```python
from build123d import *

# Parameters (mm, degrees)
MAIN_WEB_PROFILE_W                      = 60
MAIN_WEB_PROFILE_H                      = 14
MAIN_WEB_DEPTH                          = 4
SHOULDER_HORN_FLANGE_PROFILE_R          = 16
SHOULDER_HORN_FLANGE_DEPTH              = 4
ELBOW_SERVO_MOUNT_PROFILE_W             = 48
ELBOW_SERVO_MOUNT_PROFILE_H             = 28
ELBOW_SERVO_MOUNT_DEPTH                 = 4
SG90_BODY_CLEARANCE_START               = -5
SG90_BODY_CLEARANCE_PROFILE_W           = 23.8
SG90_BODY_CLEARANCE_PROFILE_H           = 13
SG90_BODY_CLEARANCE_DEPTH               = 97.49863387
ELBOW_TAB_FASTENERS_START               = -50
ELBOW_TAB_FASTENERS_PROFILE_R           = 1.3
ELBOW_TAB_FASTENERS_DEPTH               = 142.49863387
SHOULDER_CENTER_SCREW_ACCESS_START      = -50
SHOULDER_CENTER_SCREW_ACCESS_PROFILE_R  = 4
SHOULDER_CENTER_SCREW_ACCESS_DEPTH      = 142.49863387
CABLE_TIE_HOLES_START                   = -50
CABLE_TIE_HOLES_PROFILE_R               = 1.6
CABLE_TIE_HOLES_DEPTH                   = 142.49863387
PASSIVE_LOWER_MOUNT_BOSS_PROFILE_R      = 5
PASSIVE_LOWER_MOUNT_BOSS_DEPTH          = 4
PASSIVE_UPPER_MOUNT_BOSS_PROFILE_R      = 5
PASSIVE_UPPER_MOUNT_BOSS_DEPTH          = 4
PASSIVE_CHEEK_STANDOFFS_START           = -50
PASSIVE_CHEEK_STANDOFFS_PROFILE_R       = 1.6
PASSIVE_CHEEK_STANDOFFS_DEPTH           = 142.49863387
SHOULDER_DOWEL_SUPPORT_HUB_START        = 4
SHOULDER_DOWEL_SUPPORT_HUB_PROFILE_R    = 7
SHOULDER_DOWEL_SUPPORT_HUB_PROFILE_R_2  = 4
SHOULDER_DOWEL_SUPPORT_HUB_DEPTH        = 4
RAISED_M3_WASHER_SEATS_HEIGHT8_START    = 4
RAISED_M3_WASHER_SEATS_PCD14_PROFILE_R  = 3.5
RAISED_M3_WASHER_SEATS_HEIGHT8_DEPTH    = 4
METAL_HORN_M3_CLEARANCE_PCD14_START     = -50
METAL_HORN_M3_CLEARANCE_PCD14_PROFILE_R = 1.6
METAL_HORN_M3_CLEARANCE_PCD14_DEPTH     = 142.760557976
RESTORE_SHOULDER_SLEEVE_BORE_START      = -50
RESTORE_SHOULDER_SLEEVE_BORE_PROFILE_R  = 4
RESTORE_SHOULDER_SLEEVE_BORE_DEPTH      = 142.760557976
FILLET1_R                               = 7.5


with BuildPart() as part:
    # Main_web_profile → Main_web (new body)
    with BuildSketch(Plane.XY):
        with Locations((30, 0)):
            Rectangle(MAIN_WEB_PROFILE_W, MAIN_WEB_PROFILE_H)
    extrude(amount=MAIN_WEB_DEPTH)

    # Shoulder_horn_flange_profile → Shoulder_horn_flange (add)
    with BuildSketch(Plane.XY):
        Circle(SHOULDER_HORN_FLANGE_PROFILE_R)
    extrude(amount=SHOULDER_HORN_FLANGE_DEPTH)

    # Elbow_servo_mount_profile → Elbow_servo_mount (add)
    with BuildSketch(Plane.XY):
        with Locations((66, 0)):
            Rectangle(ELBOW_SERVO_MOUNT_PROFILE_W, ELBOW_SERVO_MOUNT_PROFILE_H)
    extrude(amount=ELBOW_SERVO_MOUNT_DEPTH)

    # SG90_body_clearance_profile → SG90_body_clearance (cut, through all)
    with BuildSketch(Plane.XY.offset(SG90_BODY_CLEARANCE_START)):
        with Locations((65.5, 0)):
            Rectangle(SG90_BODY_CLEARANCE_PROFILE_W, SG90_BODY_CLEARANCE_PROFILE_H)
    extrude(amount=SG90_BODY_CLEARANCE_DEPTH, mode=Mode.SUBTRACT)

    # Elbow_tab_fasteners_profile → Elbow_tab_fasteners (cut, through all)
    with BuildSketch(Plane.XY.offset(ELBOW_TAB_FASTENERS_START)):
        with Locations(Location((51, 0, 0), (0, 0, 180))):
            Circle(ELBOW_TAB_FASTENERS_PROFILE_R)
        with Locations(Location((80, 0, 0), (0, 0, 180))):
            Circle(ELBOW_TAB_FASTENERS_PROFILE_R)
    extrude(amount=ELBOW_TAB_FASTENERS_DEPTH, mode=Mode.SUBTRACT)

    # Shoulder_center_screw_access_profile → Shoulder_center_screw_access (cut, through all)
    with BuildSketch(Plane.XY.offset(SHOULDER_CENTER_SCREW_ACCESS_START)):
        with Locations(Location((0, 0, 0), (0, 0, 180))):
            Circle(SHOULDER_CENTER_SCREW_ACCESS_PROFILE_R)
    extrude(amount=SHOULDER_CENTER_SCREW_ACCESS_DEPTH, mode=Mode.SUBTRACT)

    # Cable_tie_holes_profile → Cable_tie_holes (cut, through all)
    with BuildSketch(Plane.XY.offset(CABLE_TIE_HOLES_START)):
        with Locations(Location((27, -3, 0), (0, 0, 180))):
            Circle(CABLE_TIE_HOLES_PROFILE_R)
        with Locations(Location((27, 3, 0), (0, 0, 180))):
            Circle(CABLE_TIE_HOLES_PROFILE_R)
    extrude(amount=CABLE_TIE_HOLES_DEPTH, mode=Mode.SUBTRACT)

    # Passive_lower_mount_boss_profile → Passive_lower_mount_boss (add)
    with BuildSketch(Plane.XY):
        with Locations((35, -9)):
            Circle(PASSIVE_LOWER_MOUNT_BOSS_PROFILE_R)
    extrude(amount=PASSIVE_LOWER_MOUNT_BOSS_DEPTH)

    # Passive_upper_mount_boss_profile → Passive_upper_mount_boss (add)
    with BuildSketch(Plane.XY):
        with Locations((35, 9)):
            Circle(PASSIVE_UPPER_MOUNT_BOSS_PROFILE_R)
    extrude(amount=PASSIVE_UPPER_MOUNT_BOSS_DEPTH)

    # Passive_cheek_standoffs_profile → Passive_cheek_standoffs (cut, through all)
    with BuildSketch(Plane.XY.offset(PASSIVE_CHEEK_STANDOFFS_START)):
        with Locations(Location((35, -9, 0), (0, 0, 180))):
            Circle(PASSIVE_CHEEK_STANDOFFS_PROFILE_R)
        with Locations(Location((35, 9, 0), (0, 0, 180))):
            Circle(PASSIVE_CHEEK_STANDOFFS_PROFILE_R)
    extrude(amount=PASSIVE_CHEEK_STANDOFFS_DEPTH, mode=Mode.SUBTRACT)

    # Shoulder_dowel_support_hub_profile → Shoulder_dowel_support_hub (add)
    with BuildSketch(Plane.XY.offset(SHOULDER_DOWEL_SUPPORT_HUB_START)):
        Circle(SHOULDER_DOWEL_SUPPORT_HUB_PROFILE_R)
        with Locations(Location((0, 0, 0), (0, 0, 180))):
            Circle(SHOULDER_DOWEL_SUPPORT_HUB_PROFILE_R_2, mode=Mode.SUBTRACT)
    extrude(amount=SHOULDER_DOWEL_SUPPORT_HUB_DEPTH)

    # Raised_M3_washer_seats_PCD14_profile → Raised_M3_washer_seats_height8 (add)
    with BuildSketch(Plane.XY.offset(RAISED_M3_WASHER_SEATS_HEIGHT8_START)):
        with Locations((7, 0)):
            Circle(RAISED_M3_WASHER_SEATS_PCD14_PROFILE_R)
        with Locations((-7, 0)):
            Circle(RAISED_M3_WASHER_SEATS_PCD14_PROFILE_R)
        with Locations((0, 7)):
            Circle(RAISED_M3_WASHER_SEATS_PCD14_PROFILE_R)
        with Locations((0, -7)):
            Circle(RAISED_M3_WASHER_SEATS_PCD14_PROFILE_R)
    extrude(amount=RAISED_M3_WASHER_SEATS_HEIGHT8_DEPTH)

    # Metal_horn_M3_clearance_PCD14_profile → Metal_horn_M3_clearance_PCD14 (cut, through all)
    with BuildSketch(Plane.XY.offset(METAL_HORN_M3_CLEARANCE_PCD14_START)):
        with Locations(Location((7, 0, 0), (0, 0, 180))):
            Circle(METAL_HORN_M3_CLEARANCE_PCD14_PROFILE_R)
        with Locations(Location((-7, 0, 0), (0, 0, 180))):
            Circle(METAL_HORN_M3_CLEARANCE_PCD14_PROFILE_R)
        with Locations(Location((0, 7, 0), (0, 0, 180))):
            Circle(METAL_HORN_M3_CLEARANCE_PCD14_PROFILE_R)
        with Locations(Location((0, -7, 0), (0, 0, 180))):
            Circle(METAL_HORN_M3_CLEARANCE_PCD14_PROFILE_R)
    extrude(amount=METAL_HORN_M3_CLEARANCE_PCD14_DEPTH, mode=Mode.SUBTRACT)

    # Restore_shoulder_sleeve_bore_profile → Restore_shoulder_sleeve_bore (cut, through all)
    with BuildSketch(Plane.XY.offset(RESTORE_SHOULDER_SLEEVE_BORE_START)):
        with Locations(Location((0, 0, 0), (0, 0, 180))):
            Circle(RESTORE_SHOULDER_SLEEVE_BORE_PROFILE_R)
    extrude(amount=RESTORE_SHOULDER_SLEEVE_BORE_DEPTH, mode=Mode.SUBTRACT)

    # Fillet1
    # the kernel refuses this fillet: 7.5 mm, written as the material it takes off along each edge
    with BuildSketch(Plane(origin=(42, -14, -18.708286934), x_dir=(0, 1, 0), z_dir=(0, 0, 1))) as fillet1_piece_1:
        with BuildLine():
            CenterArc((7.5, -7.483314774), FILLET1_R, 93.822553729, 86.177446271)
            Line((0, -7.483314774), (-0.15, -7.483314774))
            Line((-0.15, -7.483314774), (-0.15, 0))
            Line((-0.15, 0), (0, 0.15))
            ThreePointArc((0, 0.15), (3.5, 0.15), (6.99, 0.149666295))
            Line((6.99, 0.149666295), (7, 0))
        make_face()
    extrude(amount=41.416573868, mode=Mode.SUBTRACT)
    with BuildSketch(Plane(origin=(90, -14, -18.75), x_dir=(-1, 0, 0), z_dir=(0, 0, 1)), Plane(origin=(90, 14, -18.75), x_dir=(0, -1, 0), z_dir=(0, 0, 1))) as fillet1_piece_2:
        with BuildLine():
            CenterArc((FILLET1_R, -FILLET1_R), FILLET1_R, 90, 90)
            Line((0, -FILLET1_R), (-FILLET1_R * 0.02, -FILLET1_R))
            Line((-FILLET1_R * 0.02, -FILLET1_R), (-FILLET1_R * 0.02, FILLET1_R * 0.02))
            Line((-FILLET1_R * 0.02, FILLET1_R * 0.02), (FILLET1_R, FILLET1_R * 0.02))
            Line((FILLET1_R, FILLET1_R * 0.02), (FILLET1_R, 0))
        make_face()
    extrude(amount=41.5, mode=Mode.SUBTRACT)
    with BuildSketch(Plane(origin=(42, 14, -18.708286934), x_dir=(0, -1, 0), z_dir=(0, 0, 1))) as fillet1_piece_3:
        with BuildLine():
            CenterArc((7.5, 7.483314774), FILLET1_R, 180, 86.177446271)
            Line((0, 7.483314774), (-0.15, 7.483314774))
            Line((-0.15, 7.483314774), (-0.15, 0))
            Line((-0.15, 0), (0, -0.15))
            ThreePointArc((0, -0.15), (3.5, -0.15), (6.99, -0.149666295))
            Line((6.99, -0.149666295), (7, 0))
        make_face()
    extrude(amount=41.416573868, mode=Mode.SUBTRACT)


solid = part.part
```
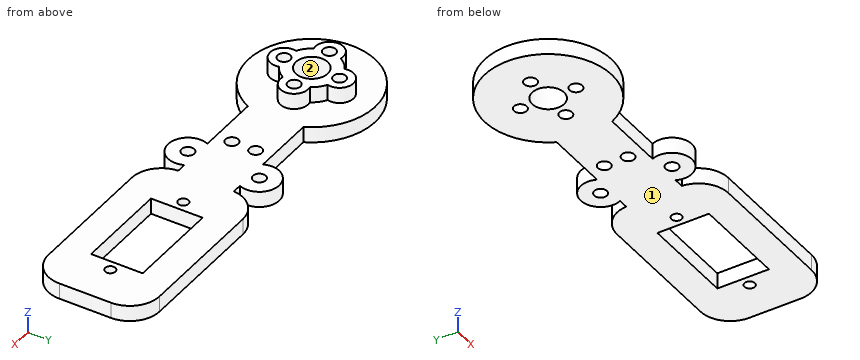
The listing builds one solid part. Answer for the finished solid, in the listing's coordinates (mm). Face numbers are marked on the shaded views. Coordinates: 2 decimals unless noted, no trailing zeros. Loops run counter-clockwise (first coordinate to the right, second up) from the corner with the lowest first, then second, coordinate; pieces in that order, holes last. Notation, with made-up numbers: M 61,35.5 L 87,35.5 A23 cw 87,46.5 Z; hole C 2.5,-10 d8. An arc over 180 degrees is marked long. Answer as a JSON object with one key per item and string values. Group by question number.
Item 1: Determine the mould class of the marked faces 1 and 2 for opening direction X: +X half, -X half, draft (parallel to the pull), parting line (faces both ways), or undercut.
Item 2: Each of these flat-tipped pins is pushed along its axis until it touches: P1, Ø3, axis at x = 0, y = -7, coming from the +Z side; P2, Ø1.2, axis at x = 64, z = 2, coming from the -Y side; P3, Ø2.5, axis at x = 40.5, z = 3, coming from the -Y side; P4, Ø4.5, axis at y = 1, z = 2.5, coming from the -X side. Where does it stop, or does it pass through?
Item 3: Section D-D (x = 0) is taken. Write down the section's boundary in (y, z), and give its area (3 significant figures).
Item 4: Section C-C (y = 0) is taken. Give the number of separate pieces and of enclosed holes in the cut face, and give its area (3 significant figures).
Item 5: Consider L1, parallel to Y at x = 0, z = 4.5; L2, parallel to X at y = -12, z = 3; L3, parallel to Y at x = 80, z = 2.65. Determine where each line is inside the solid, lowest interval first.
Item 6: Section A-A (x = 62) is taken. Write down the section's boundary in (y, z), and give its area (3 significant figures).
Item 7: Section B-B (x = 27) is taken. Write down the section's boundary in (y, z).
Solved:
{
 "1": {"face 1": "draft", "face 2": "undercut"},
 "2": {"P1": "passes through", "P2": "stops at y = -14", "P3": "stops at y = -11.63", "P4": "stops at x = -16"},
 "3": {"outline": "M -16,0 L -8.6,0 L -8.6,8 L -10.5,8 L -10.5,4 L -16,4 Z; M -5.4,0 L -4,0 L -4,8 L -5.4,8 Z; M 4,0 L 5.4,0 L 5.4,8 L 4,8 Z; M 8.6,0 L 16,0 L 16,4 L 10.5,4 L 10.5,8 L 8.6,8 Z", "area": "96.8 mm2"},
 "4": {"separate pieces": "7", "enclosed holes": "0", "area": "277 mm2"},
 "5": {"L1": "y = -10.5 to -8.6, -5.4 to -4, 4 to 5.4, 8.6 to 10.5", "L2": "x = -10.58 to 10.58, 31 to 39, 44.38 to 87.6", "L3": "y = -14 to -1.3, 1.3 to 14"},
 "6": {"outline": "M -14,0 L -6.5,0 L -6.5,4 L -14,4 Z; M 6.5,0 L 14,0 L 14,4 L 6.5,4 Z", "area": "60.0 mm2"},
 "7": {"outline": "M -7,0 L -4.6,0 L -4.6,4 L -7,4 Z; M -1.4,0 L 1.4,0 L 1.4,4 L -1.4,4 Z; M 4.6,0 L 7,0 L 7,4 L 4.6,4 Z"}
}
